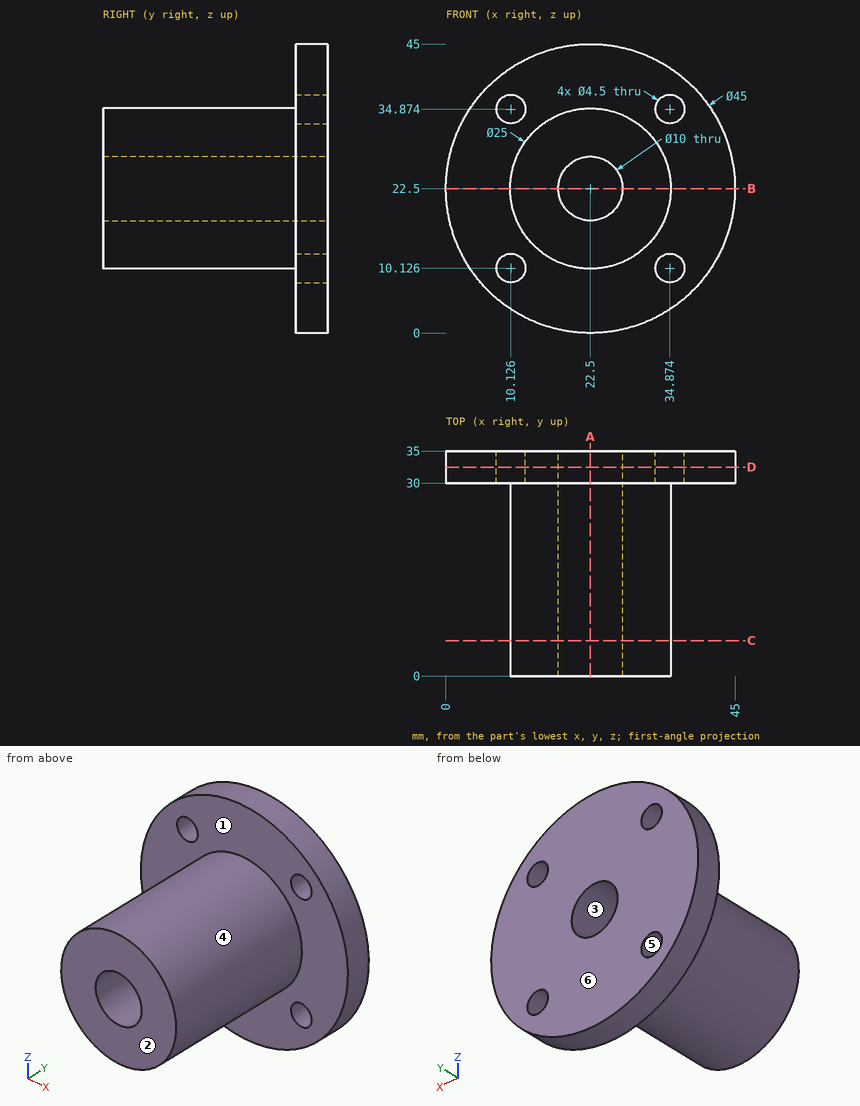
Geometry check sheet. Reference: drawing and pictorial views, mm from the part's lowest x, y, z. A direction names the side the tool comes from. Round coordinates to 2 decimals unless told otherwise and drop trailing zeros. Order: outer loops, then holes, each group sorted by start corner. A loop starts at its lowest first (then second) coordinate and runs counter-clockwise, first axis right, second up. Notation, with made-up numbers: (34, 49) - (69, 49) arc R14 cw to (69, 65) - close; hole circle Ø11 at (16.25, -15.75). An arc over 180 degrees is marked (long way). Use a Markdown table: item, result. Add a question column.
1) Mould release check, pull along Z, two halves, no side actions. Record for the marked faces 3, 4, 5 and 6: released by +Z, released by -Z, zero draft, split by the parting line, or undercut.
2) Gauge pin test, flat ends, axial feed: P1, Ø3, axis at y = 13, z = 28.5, coming from the +X side; P2, Ø3, axis at x = 14.5, y = 5, coming from the -Z side; P3, Ø12, axis at x = 37.5, z = 36, coming from the -Y side. Record the tip position at first contact, or that the pin passes through.
3) Section check D-D (y = 32.5). Count the separate pieces of the cut face and the enclosed holes in it, then the cut area to 3 significant figures.
4) Set-up check for the marked faces 1 and 2: record each of +Z, -Z, +X, -X, +Y, -Y from which the full face is reachable in a straight line by a thin tool's end or side.
5) Section check A-A (x = 22.5). Record the cut outline in (y, z), then the cut area to 3 significant figures.
6) Section check C-C (y = 5.5). Record the cut outline in (x, z).
7) Section check B-B (z = 22.5). Record the cut outline in (x, y), then the cut area to 3 significant figures.
8) Thickness scan on line 1 along X through (y, z) = (14.5, 22.5); line 2 along Z through (x, y) = (26.5, 30.5); line 3 along Y through (x, z) = (28, 9). Record the ranges inside material, lowest first.
Established:
| question | item | result |
|---|---|---|
| 1 | face 3 | undercut |
| 1 | face 4 | split by the parting line |
| 1 | face 5 | undercut |
| 1 | face 6 | zero draft |
| 2 | P1 | x = 34.16 |
| 2 | P2 | z = 11.82 |
| 2 | P3 | y = 30 |
| 3 | separate pieces | 1 |
| 3 | enclosed holes | 5 |
| 3 | area | 1,450 mm2 |
| 4 | face 1 | -Y |
| 4 | face 2 | +Z, -Z, +X, -X, -Y |
| 5 | outline | (0, 10) - (30, 10) - (30, 0) - (35, 0) - (35, 17.5) - (0, 17.5) - close; (0, 27.5) - (35, 27.5) - (35, 45) - (30, 45) - (30, 35) - (0, 35) - close |
| 5 | area | 625 mm2 |
| 6 | outline | circle Ø25 at (22.5, 22.5); hole circle Ø10 at (22.5, 22.5) |
| 7 | outline | (0, 30) - (10, 30) - (10, 0) - (17.5, 0) - (17.5, 35) - (0, 35) - close; (27.5, 0) - (35, 0) - (35, 30) - (45, 30) - (45, 35) - (27.5, 35) - close |
| 7 | area | 625 mm2 |
| 8 | line 1 | 10 to 17.5, 27.5 to 35 |
| 8 | line 2 | 0.36 to 19.5, 25.5 to 44.64 |
| 8 | line 3 | 30 to 35 |
